The drawing under review shows one solid part. Ordinate dimensions are in mm from its lowest x, y, z. A direction names the side the tool comes from. Round coordinates to 2 decimals unless told otherwise and drop trailing zeros. Order: outer loops, then holes, each group sorted by start corner. A loop starts at its lowest first (then second) coordinate and runs counter-clockwise, first axis right, second up. Notation, with made-up numbers: M 34.25,-1 L 86.25,-1 A12 cw 86.25,20 Z; hole C 20.5,70.25 d5. An arc over 180 degrees is marked long. Answer as a JSON object with one key per item and string values. Group by question number.
1) Consider section B-B, the plane z = 9.5. Write out the cut boundary in (x, y), then the cut area to 3 significant figures.
2) Insertion check: pin 1 Ø0.7 at (x, y) = (12, 1) entering from +Z; pin 2 Ø1.1 at (y, z) = (0.5, 8.5) entering from +X; pin 3 Ø9 at (x, z) = (12, 10) entering from -Y; pin 4 Ø1.5 at (x, y) = (12, 0.5) entering from -Z. Each pin has a flat end and moves straight along its axis. Give the tip position at first contact, or say it passes through.
3) Consider section A-A, the plane y = 4.25. Write out the cut boundary in (x, z), then the cut area to 3 significant figures.
4) Consider section C-C, the plane x = 2.54. Write out the cut boundary in (y, z).
5) For the marked faces 1 and 2, list the 3-axis set-ups (+Z, -Z, +X, -X, +Y, -Y) from which the entire face can be reached by the end or side of a thin tool; tool diameter is ignored.
6) To check wall thickness, follow line 1 (Y direction, x = 4, z = 5.5); line 2 (X direction, y = 1, z = 8); line 3 (X direction, y = 5.65, z = 16.5). State the ranges of each line that lie inside material, in increasing order.
7) Consider section D-D, the plane x = 20. Write out the cut boundary in (y, z), then the cut area to 3 significant figures.
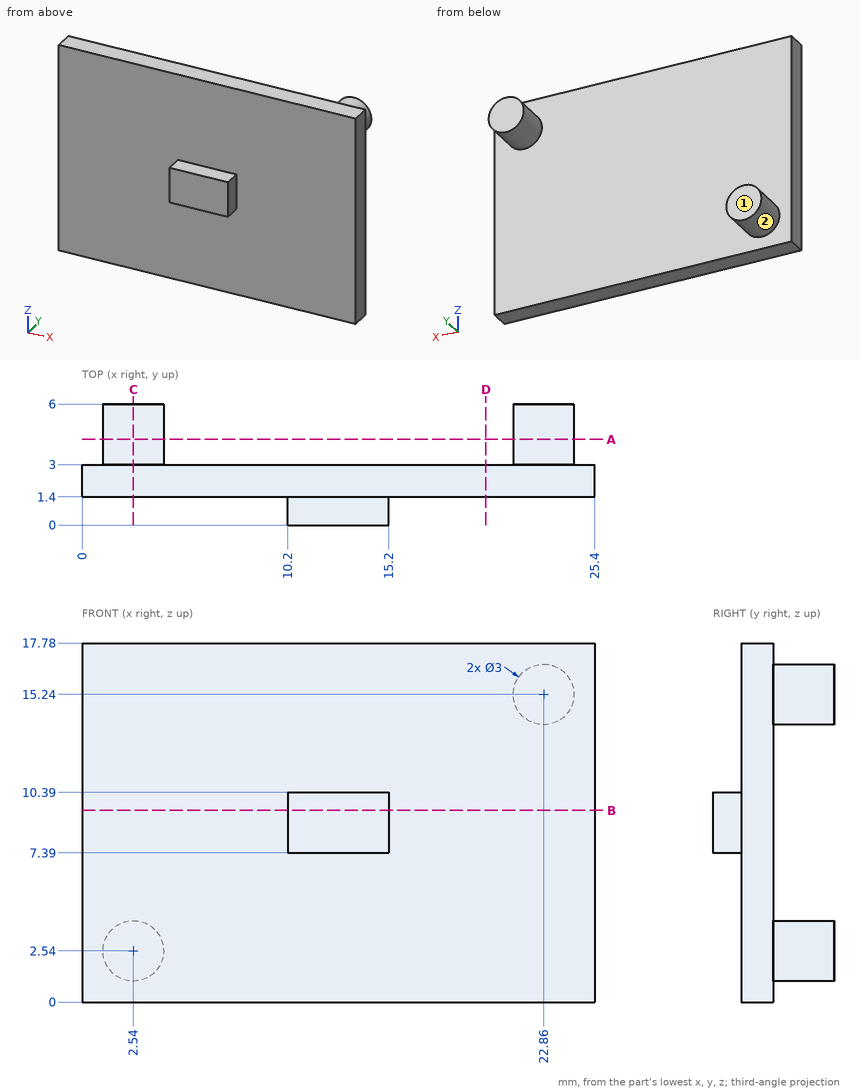
Results list:
{
 "1": {"outline": "M 0,1.4 L 10.2,1.4 L 10.2,0 L 15.2,0 L 15.2,1.4 L 25.4,1.4 L 25.4,3 L 0,3 Z", "area": "47.6 mm^2"},
 "2": {"pin 1": "z = 10.39", "pin 2": "x = 15.2", "pin 3": "y = 0", "pin 4": "z = 7.39"},
 "3": {"outline": "C 2.54,2.54 d3; C 22.86,15.24 d3", "area": "14.1 mm^2"},
 "4": {"outline": "M 1.4,0 L 3,0 L 3,1.04 L 6,1.04 L 6,4.04 L 3,4.04 L 3,17.78 L 1.4,17.78 Z"},
 "5": {"face 1": "+Z, -Z, +X, -X, +Y", "face 2": "+Y"},
 "6": {"line 1": "1.4 to 3", "line 2": "10.2 to 15.2", "line 3": "22.05 to 23.67"},
 "7": {"outline": "M 1.4,0 L 3,0 L 3,17.78 L 1.4,17.78 Z", "area": "28.4 mm^2"}
}
